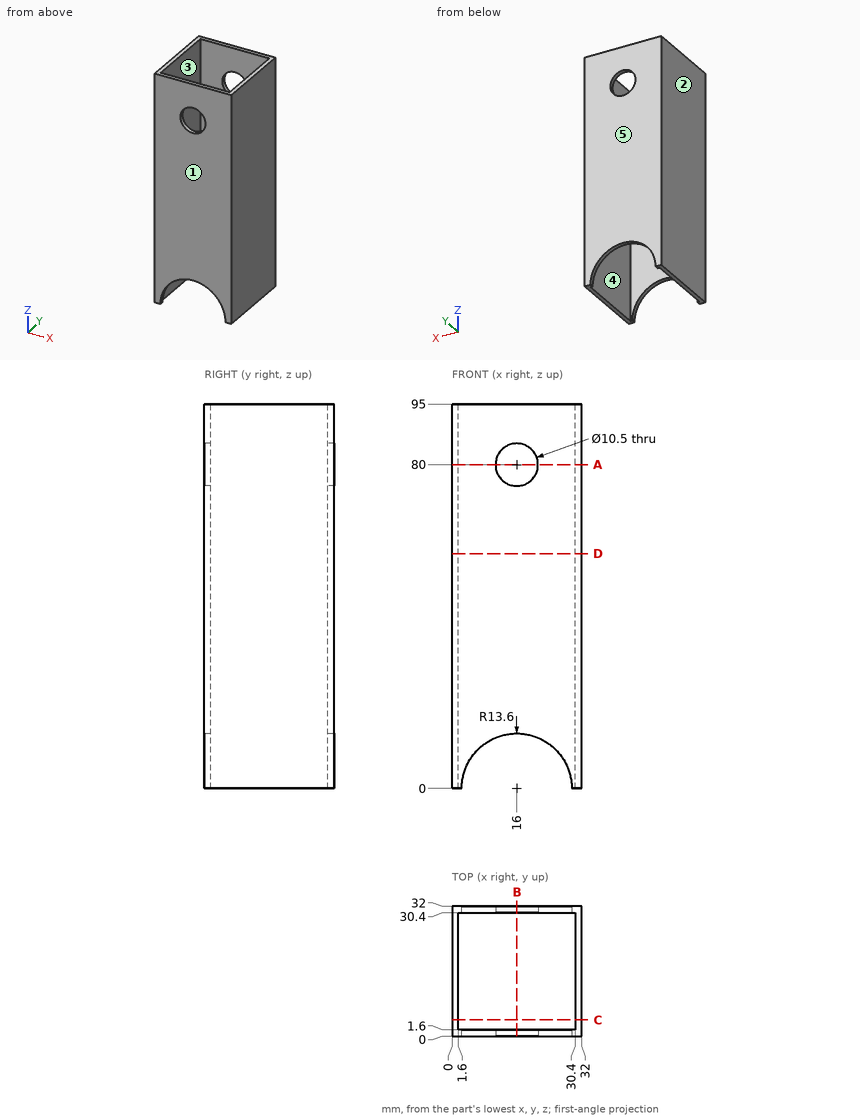
Design review of the part shown in the three views and the two pictorial views. Dimensions are in mm from the part's minimum x, y and z. A direction names the side the tool comes from. Round coordinates to 2 decimals unless told otherwise and drop trailing zeros. Loops run counter-clockwise (first coordinate to the right, second up) from the corner with the lowest first, then second, coordinate; pieces in that order, holes last. Notation, with made-up numbers: (64.5, 68) - (76.5, 68) arc R23 cw to (76.5, 76) - close; hole circle Ø5 at (-20.5, 14.25). An arc over 180 degrees is marked (long way). Write each question's results on one line, items separated by ' | '. Start each with the question number.
Q1. Wall thickness on line 1 along Y through (x, z) = (23, 63.5); line 2 along X through (y, z) = (1, 80): over which ranges is each line inside the solid? List them lowest first. Write a range as [from, to].
Q2. Take a section at D-D on z = 58. Give the boundary of the cut face in (x, y).
Q3. Take a section at C-C on y = 4. Give the boundary of the cut face in (x, z).
Q4. Tool access review of the marked faces 4 and 5: name each direction out of +Z, -Z, +X, -X, +Y, -Y from which nothing blocks a thin tool from reaching the whole face with its end or side.
Q5. Take a section at A-A on z = 80. Give the boundary of the cut face in (x, y).
Q6. Take a section at B-B on x = 16. Give the boundary of the cut face in (y, z), plus the area to 3 significant figures.
Q7. Draft analysis for pull direction X (two halves, no side actions). For the marked faces 1, 2 and 3, state which applies: pulls with the +X half, pulls with the -X half, needs draft (parallel to the pull), parting line crosses it, or undercut.
Data:
1) line 1: y = [0, 1.6], [30.4, 32] | line 2: x = [0, 10.75], [21.25, 32]
2) outline: (0, 0) - (32, 0) - (32, 32) - (0, 32) - close; hole (1.6, 1.6) - (30.4, 1.6) - (30.4, 30.4) - (1.6, 30.4) - close
3) outline: (0, 0) - (1.6, 0) - (1.6, 95) - (0, 95) - close; (30.4, 0) - (32, 0) - (32, 95) - (30.4, 95) - close
4) face 4: +Z, -Z | face 5: +Z, -Z, +X, -X, +Y
5) outline: (0, 0) - (10.75, 0) - (10.75, 1.6) - (1.6, 1.6) - (1.6, 30.4) - (10.75, 30.4) - (10.75, 32) - (0, 32) - close; (21.25, 0) - (32, 0) - (32, 32) - (21.25, 32) - (21.25, 30.4) - (30.4, 30.4) - (30.4, 1.6) - (21.25, 1.6) - close
6) outline: (0, 13.6) - (1.6, 13.6) - (1.6, 74.75) - (0, 74.75) - close; (0, 85.25) - (1.6, 85.25) - (1.6, 95) - (0, 95) - close; (30.4, 13.6) - (32, 13.6) - (32, 74.75) - (30.4, 74.75) - close; (30.4, 85.25) - (32, 85.25) - (32, 95) - (30.4, 95) - close | area: 227 mm²
7) face 1: needs draft | face 2: pulls with the -X half | face 3: undercut
